```python
from build123d import *

# Parameters (mm, degrees)
SKETCH1_R           = 18.75
BOSS_EXTRUDE1_DEPTH = 7
SKETCH2_R           = 1.5
CUT_EXTRUDE1_DEPTH  = 7
SKETCH3_R           = 21.75
SKETCH3_R_2         = 13
BOSS_EXTRUDE2_DEPTH = 0.8
SKETCH5_W           = 3.633456263
SKETCH5_H           = 7
BOSS_EXTRUDE4_DEPTH = 15
BOSS_EXTRUDE5_DEPTH = 7
SKETCH7_R           = 1.5
CUT_EXTRUDE2_DEPTH  = 6
SKETCH8_W           = 8.171206901
SKETCH8_H           = 6.05024239
BOSS_EXTRUDE6_DEPTH = 8
SKETCH9_R           = 1.5
CUT_EXTRUDE3_DEPTH  = 10
FILLET1_R           = 2


with BuildPart() as part:
    # Sketch1 → Boss-Extrude1 (new body)
    with BuildSketch(Plane(origin=(0, 0, 0), x_dir=(1, 0, 0), z_dir=(0, 1, 0))):
        with BuildLine():
            Line((3.5, -25.1), (-3.5, -25.1))
            Line((-3.5, -25.1), (-3.5, -21.466543737))
            ThreePointArc((-3.5, -21.466543737), (0, 21.75), (3.5, -21.466543737))
            Line((3.5, -21.466543737), (3.5, -25.1))
        make_face()
        Circle(SKETCH1_R, mode=Mode.SUBTRACT)
    extrude(amount=BOSS_EXTRUDE1_DEPTH)

    # Sketch2 → Cut-Extrude1 (cut)
    with BuildSketch(Plane.XY.offset(25.1)):
        with Locations((0, 3.5)):
            Circle(SKETCH2_R)
    extrude(amount=-CUT_EXTRUDE1_DEPTH, mode=Mode.SUBTRACT)

    # Sketch3 → Boss-Extrude2 (add)
    with BuildSketch(Plane.XZ):
        Circle(SKETCH3_R)
        Circle(SKETCH3_R_2, mode=Mode.SUBTRACT)
    extrude(amount=BOSS_EXTRUDE2_DEPTH)

    # Sketch5 → Boss-Extrude4 (add)
    with BuildSketch(Plane(origin=(3.5, 0, 0), x_dir=(0, 0, -1), z_dir=(1, 0, 0))):
        with Locations((-23.283271869, 3.5)):
            Rectangle(SKETCH5_W, SKETCH5_H)
    extrude(amount=BOSS_EXTRUDE4_DEPTH)

    # Sketch6 → Boss-Extrude5 (add)
    with BuildSketch(Plane(origin=(0, 7, 0), x_dir=(1, 0, 0), z_dir=(0, 1, 0))):
        Polygon((18.5, -25.1), (18.5, -11.437329234), (3.5, -21.466543737), (3.5, -25.1), align=None)
    extrude(amount=-BOSS_EXTRUDE5_DEPTH)

    # Sketch7 → Cut-Extrude2 (cut)
    with BuildSketch(Plane.XY.offset(25.1)):
        with Locations((10, 3.5)):
            Circle(SKETCH7_R)
    extrude(amount=-CUT_EXTRUDE2_DEPTH, mode=Mode.SUBTRACT)

    # Sketch8 → Boss-Extrude6 (add)
    with BuildSketch(Plane(origin=(0, 7, 0), x_dir=(1, 0, 0), z_dir=(0, 1, 0))):
        with Locations((0.585603451, -22.074878805)):
            Rectangle(SKETCH8_W, SKETCH8_H)
    extrude(amount=BOSS_EXTRUDE6_DEPTH)

    # Sketch9 → Cut-Extrude3 (cut)
    with BuildSketch(Plane.XY.offset(25.1)):
        with Locations((0, 11.5)):
            Circle(SKETCH9_R)
    extrude(amount=-CUT_EXTRUDE3_DEPTH, mode=Mode.SUBTRACT)

    # Fillet1
    fillet1_edges = [part.edges().sort_by_distance(p)[0] for p in [
        (-3.5, 15, 22.074878805),
        (4.671206901, 15, 22.074878805),
    ]]
    fillet(fillet1_edges, radius=FILLET1_R)


solid = part.part
```
Can you work these out from the model? Positions are in its coordinate system, mm. A direction names the side the tool comes from. Give positions to 0.01 mm unless a question says otherwise; leave off trailing zeros. Order: outer loops, then holes, each group sorted by start corner. A loop starts at its lowest first (then second) coordinate and runs counter-clockwise, first axis right, second up. Notation, with made-up numbers: M -20,-11.75 L 22,-11.75 A21 cw 22,24.25 Z; hole C 56,78.5 d2. An arc over 180 degrees is marked long. One line per item, written item: value.
1) For P1, Ø13, axis at x = -7, z = -4, coming from the +Y side; P2, Ø6, axis at y = 12.5, z = -1.5, coming from the +X side; P3, Ø2.5, axis at x = -1, y = 12.5, coming from the -Z side; P4, Ø3, axis at y = 11.5, z = 21.5, coming from the +X side, each with a flat end and sliding along its axis, tell me the tip position at first contact or that it passes through.
Answer sheet:
P1: stops at y = 0
P2: passes through
P3: stops at z = 19.05
P4: stops at x = 4.67
2) I want a section at C-C, the plane z = 0. List the corners of the cut face in (x, y) for me, plus the area to 3 significant figures.
Answer sheet:
outline: M -21.75,-0.8 L -13,-0.8 L -13,0 L -18.75,0 L -18.75,7 L -21.75,7 Z; M 13,-0.8 L 21.75,-0.8 L 21.75,7 L 18.75,7 L 18.75,0 L 13,0 Z
area: 56.0 mm^2
3) I want a section at A-A, the plane x = 0. List the corners of the cut face in (y, z) for me.
Answer sheet:
outline: M -0.8,-21.75 L 7,-21.75 L 7,-18.75 L 0,-18.75 L 0,-13 L -0.8,-13 Z; M -0.8,13 L 0,13 L 0,18.75 L 2,18.75 L 2,25.1 L 0,25.1 L 0,21.75 L -0.8,21.75 Z; M 5,18.75 L 7,18.75 L 7,19.05 L 10,19.05 L 10,25.1 L 5,25.1 Z; M 13,19.05 L 15,19.05 L 15,25.1 L 13,25.1 Z
4) I want a section at D-D, the plane y = 3.5. List the corners of the cut face in (x, z) for me, plus the area to 3 significant figures.
Answer sheet:
outline: M -3.5,21.47 A21.75 ccw long 18.5,11.44 L 18.5,25.1 L 11.5,25.1 L 11.5,19.1 L 8.5,19.1 L 8.5,25.1 L 1.5,25.1 L 1.5,18.69 A18.75 cw long -1.5,18.69 L -1.5,25.1 L -3.5,25.1 Z
area: 475 mm^2
5) Please list where these lines run through material, in increasing order: line 1 along Y through (x, z) = (0, 22); line 2 along X through (y, z) = (1.5, 0); line 3 along Z through (x, y) = (0, -0.3).
Answer sheet:
line 1: y = 0 to 2, 5 to 10, 13 to 15
line 2: x = -21.75 to -18.75, 18.75 to 21.75
line 3: z = -21.75 to -13, 13 to 21.75
6) We'd pull the mould along Y, two halves only. Please class faces 5 (the face through (4.1, 14.4, 22)), 6 (the face through (8.5, 3.57, 22.14)), 7 (the face through (1, 10, 19.05)): released by +Y, released by -Y, zero draft, split by the parting line, or undercut.
Answer sheet:
face 5: released by +Y
face 6: undercut
face 7: zero draft
7) I want a section at B-B, the plane y = 11.5. List the corners of the cut face in (x, z) for me.
Answer sheet:
outline: M -3.5,19.05 L -1.5,19.05 L -1.5,25.1 L -3.5,25.1 Z; M 1.5,19.05 L 4.67,19.05 L 4.67,25.1 L 1.5,25.1 Z
8) On a 3-axis mill with a long thin cutter (end or side, diameter ignored), from which of +Z, -Z, +X, -X, +Y, -Y can I reach the whole of each face in a straight line? I mean faces 1 (the face through (4.671, 10, 22)), 2 (the face through (-3.5, 8, 23)), 3 (the face through (10, 4, 19.1)), 4 (the face through (4, 0, 13)). Say none if no direction works.
Answer sheet:
face 1: +Z, -Z, +X, +Y
face 2: +Z, -X, +Y
face 3: +Z
face 4: +Y
